Input: part model. Units: mm. Frame: model coordinates. Face numbers are marked on the shaded views. Give positions to 0.01 mm unless a question says otherwise; leave off trailing zeros. Loops run counter-clockwise (first coordinate to the right, second up) from the corner with the lowest first, then second, coordinate; pieces in that order, holes last. Notation, with made-up numbers: (-38.5, 49) - (-20.5, 49) arc R21 cw to (-20.5, 56) - close; hole circle Ø11 at (44.25, -16.75). An arc over 180 degrees is marked (long way). One line per item, written item: value.
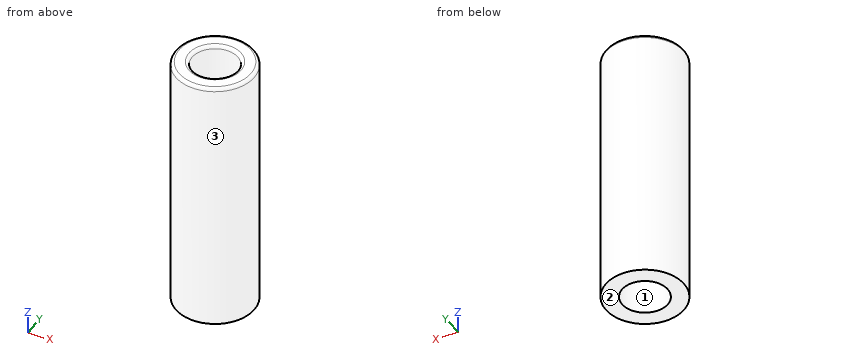
from build123d import *

# Parameters (mm, degrees)
SZKIC1_R                    = 6
SZKIC1_R_2                  = 3.5
DODANIE_WYCI_GNI_CIE1_DEPTH = 40
ZAOKR_GLENIE1_R             = 0.5
ZAOKR_GLENIE2_R             = 0.5


with BuildPart() as part:
    # Szkic1 → Dodanie-wyciągnięcie1 (new body)
    with BuildSketch(Plane.XY):
        Circle(SZKIC1_R)
        Circle(SZKIC1_R_2, mode=Mode.SUBTRACT)
    extrude(amount=DODANIE_WYCI_GNI_CIE1_DEPTH)

    # Zaokrąglenie1
    zaokr_glenie1_edges = [part.edges().sort_by_distance(p)[0] for p in [
        (-6, 0, 40),
    ]]
    fillet(zaokr_glenie1_edges, radius=ZAOKR_GLENIE1_R)

    # Zaokrąglenie2
    zaokr_glenie2_edges = [part.edges().sort_by_distance(p)[0] for p in [
        (-3.5, 0, 40),
    ]]
    fillet(zaokr_glenie2_edges, radius=ZAOKR_GLENIE2_R)


solid = part.part
Item 1: Pin query (flat end, axial travel): P1, Ø3, axis at y = -2, z = 23, coming from the -X side; P2, Ø1.5, axis at x = 1.5, z = 19, coming from the +Y side; P3, Ø1.5, axis at y = -3, z = 18.5, coming from the -X side. Return the tip coordinate at first contact, or that it passes through.
Verdict:
P1: stops at x = -5.98
P2: stops at y = 5.95
P3: stops at x = -5.56
Item 2: Section C-C, the plane z = 31.5. Output: boundary loops of the cut face in (x, y), and give its area (3 significant figures).
Verdict:
outline: circle Ø12 at (0, 0); hole circle Ø7 at (0, 0)
area: 74.6 mm^2
Item 3: Material intervals for L1, parallel to Y at x = 0, z = 27.5; L2, parallel to Y at x = -0.75, z = 25; L3, parallel to X at y = 3.75, z = 3, sorted ascending.
Verdict:
L1: y = -6 to -3.5, 3.5 to 6
L2: y = -5.95 to -3.42, 3.42 to 5.95
L3: x = -4.68 to 4.68
Item 4: Section A-A, the plane y = 0. Output: boundary loops of the cut face in (x, z), and give its area (3 significant figures).
Verdict:
outline: (-6, 0) - (-3.5, 0) - (-3.5, 39.5) arc R0.5 ccw to (-4, 40) - (-5.5, 40) arc R0.5 ccw to (-6, 39.5) - close; (3.5, 0) - (6, 0) - (6, 39.5) arc R0.5 ccw to (5.5, 40) - (4, 40) arc R0.5 ccw to (3.5, 39.5) - close
area: 200 mm^2
Item 5: Draft query along X for the marked faces 1, 2 and 3. Return one class per face: pulls with the +X half, pulls with the -X half, needs draft (parallel to the pull), parting line crosses it, or undercut.
Verdict:
face 1: undercut
face 2: needs draft
face 3: parting line crosses it
